The drawing under review shows one solid part. Ordinate dimensions are in mm from its lowest x, y, z. Round coordinates to 2 decimals unless told otherwise and drop trailing zeros. Order: outer loops, then holes, each group sorted by start corner. A loop starts at its lowest first (then second) coordinate and runs counter-clockwise, first axis right, second up. Notation, with made-up numbers: (47.25, 7.5) -> (67.25, 7.5) arc R31 cw to (67.25, 40.5) -> close; hole circle Ø7 at (14, 8). An arc over 180 degrees is marked (long way). Use a Markdown table: item, result. Add a question column.
1) Wall thickness on line 1 along X through (y, z) = (15.5, 1); line 2 along Y through (x, z) = (86.5, 0.25) (1 decimal); line 3 along Y through (x, z) = (4.5, 1): over which ranges is each line inside the solid? List them lowest first. Write a range as [from, to].
2) Consider section A-A (x = 4.5). State the section outline as (y, z) points.
3) Consider section B-B (y = 15.5). State the section outline as (x, z) points, plus the area to 3 significant figures.
4) Consider section C-C (z = 0.4). State the section outline as (x, y) points, plus the area to 3 significant figures.
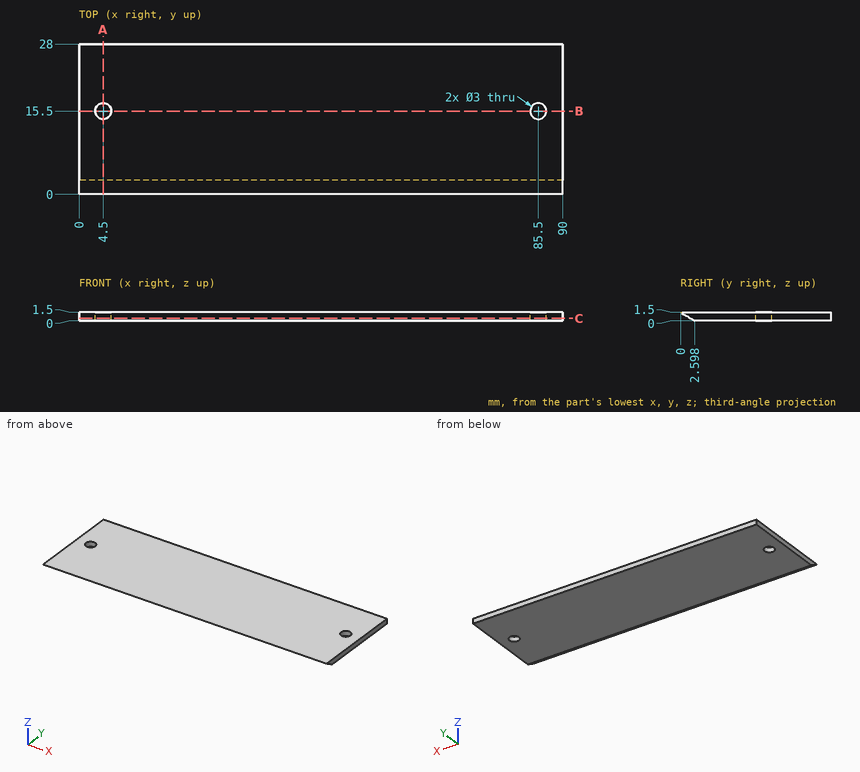
Results list:
| question | item | result |
|---|---|---|
| 1 | line 1 | [0, 3], [6, 84], [87, 90] |
| 1 | line 2 | [2.2, 14.4], [16.6, 28] |
| 1 | line 3 | [0.87, 14], [17, 28] |
| 2 | outline | (0, 1.5) -> (2.6, 0) -> (14, 0) -> (14, 1.5) -> close; (17, 0) -> (28, 0) -> (28, 1.5) -> (17, 1.5) -> close |
| 3 | outline | (0, 0) -> (3, 0) -> (3, 1.5) -> (0, 1.5) -> close; (6, 0) -> (84, 0) -> (84, 1.5) -> (6, 1.5) -> close; (87, 0) -> (90, 0) -> (90, 1.5) -> (87, 1.5) -> close |
| 3 | area | 126 mm2 |
| 4 | outline | (0, 1.91) -> (90, 1.91) -> (90, 28) -> (0, 28) -> close; hole circle Ø3 at (4.5, 15.5); hole circle Ø3 at (85.5, 15.5) |
| 4 | area | 2,330 mm2 |
